For this review, take the finished solid that the model builds, in its own axes (mm). Face numbers are marked on the shaded views. Give positions to 0.01 mm unless a question says otherwise; leave off trailing zeros. Loops run counter-clockwise (first coordinate to the right, second up) from the corner with the lowest first, then second, coordinate; pieces in that order, holes last.
```python
from build123d import *
from OCP.BRepFilletAPI import BRepFilletAPI_MakeChamfer

# Parameters (mm, degrees)
SKETCH1_W            = 68.5
SKETCH1_H            = 64.5
BOSS_EXTRUDE3_DEPTH  = 21
SKETCH3_W            = 60.5
SKETCH3_H            = 60.5
CUT_EXTRUDE1_DEPTH   = 15
SKETCH5_W            = 68.5
SKETCH5_H            = 6
BOSS_EXTRUDE4_DEPTH  = 105
SKETCH10_W           = 10
SKETCH10_H           = 29
BOSS_EXTRUDE5_DEPTH  = 5.5
SKETCH9_W            = 4
SKETCH9_H            = 20
CUT_EXTRUDE2_DEPTH   = 20.5
SKETCH11_W           = 6
SKETCH11_H           = 20
CUT_EXTRUDE3_DEPTH   = 5.5
CHAMFER2_SIZE        = 5.5
CHAMFER2_SIZE_2      = 5
CHAMFER3_SIZE        = 2
SKETCH12_W           = 34.25
SKETCH12_H           = 169.5
CUT_EXTRUDE4_DEPTH   = 50
SKETCH15_R           = 1.5
CUT_EXTRUDE5_DEPTH   = 50
SKETCH16_R           = 1.5
CUT_EXTRUDE6_DEPTH   = 50
SKETCH17_R           = 1.5
CUT_EXTRUDE7_DEPTH   = 50
SKETCH19_W           = 34.25
SKETCH19_H           = 6
BOSS_EXTRUDE6_DEPTH  = 7
SKETCH26_W           = 12
SKETCH26_H           = 9
BOSS_EXTRUDE7_DEPTH  = 30
SKETCH20_R           = 3.75
CUT_EXTRUDE9_DEPTH   = 184.263642057
SKETCH21_W           = 3
SKETCH21_H           = 2.563068229
CUT_EXTRUDE10_DEPTH  = 184.263642057
SKETCH18_R           = 1.5
CUT_EXTRUDE8_DEPTH   = 135
SKETCH24_R           = 4
CUT_EXTRUDE13_DEPTH  = 183.278118544
SKETCH25_W           = 3
SKETCH25_H           = 2.291900756
CUT_EXTRUDE14_DEPTH  = 183.278118544
SKETCH27_R           = 1.75
CUT_EXTRUDE15_DEPTH  = 183.278118544
BOSS_EXTRUDE9_START  = 5
SKETCH30_W           = 8
SKETCH30_H           = 8
SKETCH30_R           = 1.75
BOSS_EXTRUDE9_DEPTH  = 5
SKETCH31_W           = 8
SKETCH31_H           = 8
CUT_EXTRUDE16_DEPTH  = 5
SKETCH32_W           = 19.705511252
SKETCH32_H           = 22.257631466
BOSS_EXTRUDE10_DEPTH = 6
SKETCH33_R           = 1.5
CUT_EXTRUDE17_DEPTH  = 9.74
SKETCH34_R           = 3.75
CUT_EXTRUDE18_DEPTH  = 192.688549475
SKETCH36_R           = 2.5
CUT_EXTRUDE20_DEPTH  = 2
SKETCH39_W           = 3
SKETCH39_H           = 4.259893973
CUT_EXTRUDE22_DEPTH  = 192.688549475
SKETCH41_W           = 12
SKETCH41_H           = 9
BOSS_EXTRUDE11_DEPTH = 30
SKETCH42_R           = 3
CUT_EXTRUDE23_DEPTH  = 3
SKETCH44_W           = 10
SKETCH44_H           = 10
BOSS_EXTRUDE12_DEPTH = 5
SKETCH47_R           = 2.5
CUT_EXTRUDE26_DEPTH  = 3
SKETCH46_W           = 4
SKETCH46_H           = 9
CUT_EXTRUDE27_DEPTH  = 9
CUT_EXTRUDE28_START  = -68.5
SKETCH48_R           = 1.5
CUT_EXTRUDE28_DEPTH  = 68.5


with BuildPart() as part:
    # Sketch1 → Boss-Extrude3 (new body)
    with BuildSketch(Plane(origin=(0, 0, 0), x_dir=(1, 0, 0), z_dir=(0, 1, 0))):
        with Locations((-34.25, 32.25)):
            Rectangle(SKETCH1_W, SKETCH1_H)
    extrude(amount=BOSS_EXTRUDE3_DEPTH)

    # Sketch3 → Cut-Extrude1 (cut)
    with BuildSketch(Plane(origin=(0, 21, 0), x_dir=(1, 0, 0), z_dir=(0, 1, 0))):
        with Locations((-34.25, 34.25)):
            Rectangle(SKETCH3_W, SKETCH3_H)
    extrude(amount=-CUT_EXTRUDE1_DEPTH, mode=Mode.SUBTRACT)

    # Sketch5 → Boss-Extrude4 (add)
    with BuildSketch(Plane(origin=(0, 0, -64.5), x_dir=(-1, 0, 0), z_dir=(0, 0, -1))):
        with Locations((34.25, 3)):
            Rectangle(SKETCH5_W, SKETCH5_H)
    extrude(amount=BOSS_EXTRUDE4_DEPTH)

    # Sketch10 → Boss-Extrude5 (add)
    with BuildSketch(Plane.XZ):
        with Locations((-5, -30)):
            Rectangle(SKETCH10_W, SKETCH10_H)
    extrude(amount=BOSS_EXTRUDE5_DEPTH)

    # Sketch9 → Cut-Extrude2 (cut)
    with BuildSketch(Plane(origin=(0, 21, 0), x_dir=(1, 0, 0), z_dir=(0, 1, 0))):
        with Locations((-2, 28)):
            Rectangle(SKETCH9_W, SKETCH9_H)
    extrude(amount=-CUT_EXTRUDE2_DEPTH, mode=Mode.SUBTRACT)

    # Sketch11 → Cut-Extrude3 (cut)
    with BuildSketch(Plane(origin=(0, 6, 0), x_dir=(1, 0, 0), z_dir=(0, 1, 0))):
        with Locations((-7, 28)):
            Rectangle(SKETCH11_W, SKETCH11_H)
    extrude(amount=-CUT_EXTRUDE3_DEPTH, mode=Mode.SUBTRACT)

    # Chamfer2
    chamfer2_edges_1 = [part.edges().sort_by_distance(p)[0] for p in [
        (-5, -5.5, -44.5),
    ]]
    chamfer2_side_1 = [part.faces().sort_by_distance(p)[0] for p in [
        (-5, -5.4, -44.5),
    ]]
    chamfer2_edges_2 = [part.edges().sort_by_distance(p)[0] for p in [
        (-5, -5.5, -15.5),
    ]]
    chamfer2_side_2 = [part.faces().sort_by_distance(p)[0] for p in [
        (-5, -5.5, -15.6),
    ]]
    chamfer2 = BRepFilletAPI_MakeChamfer(part.part.solid().wrapped)
    for e in chamfer2_edges_1:
        chamfer2.Add(CHAMFER2_SIZE - 0.0001, CHAMFER2_SIZE_2 - 0.0001, e.wrapped, chamfer2_side_1[0].wrapped)
    for e in chamfer2_edges_2:
        chamfer2.Add(CHAMFER2_SIZE_2 - 0.0001, CHAMFER2_SIZE - 0.0001, e.wrapped, chamfer2_side_2[0].wrapped)
    add(Compound.cast(chamfer2.Shape()), mode=Mode.REPLACE)  # a hair under: the kernel refuses the full size

    # Chamfer3
    chamfer3_edges = [part.edges().sort_by_distance(p)[0] for p in [
        (-5, 0.5, -38),
        (-5, 0.5, -18),
    ]]
    chamfer(chamfer3_edges, length=CHAMFER3_SIZE)

    # Sketch12 → Cut-Extrude4 (cut)
    with BuildSketch(Plane(origin=(0, 21, 0), x_dir=(1, 0, 0), z_dir=(0, 1, 0))):
        with Locations((-51.375, 84.75)):
            Rectangle(SKETCH12_W, SKETCH12_H)
    extrude(amount=-CUT_EXTRUDE4_DEPTH, mode=Mode.SUBTRACT)

    # Sketch15 → Cut-Extrude5 (cut)
    with BuildSketch(Plane(origin=(0, 0.5, 0), x_dir=(1, 0, 0), z_dir=(0, 1, 0))):
        with Locations(Location((-5, 31.75713966, 0), (0, 0, 270))):
            Circle(SKETCH15_R)
    extrude(amount=-CUT_EXTRUDE5_DEPTH, mode=Mode.SUBTRACT)

    # Sketch16 → Cut-Extrude6 (cut)
    with BuildSketch(Plane(origin=(0, 6, 0), x_dir=(1, 0, 0), z_dir=(0, 1, 0))):
        with Locations(Location((-6, 6, 0), (0, 0, 270))):
            Circle(SKETCH16_R)
    extrude(amount=-CUT_EXTRUDE6_DEPTH, mode=Mode.SUBTRACT)

    # Sketch17 → Cut-Extrude7 (cut)
    with BuildSketch(Plane(origin=(0, 6, 0), x_dir=(1, 0, 0), z_dir=(0, 1, 0))):
        with Locations(Location((-6, 62.5, 0), (0, 0, 270))):
            Circle(SKETCH17_R)
    extrude(amount=-CUT_EXTRUDE7_DEPTH, mode=Mode.SUBTRACT)

    # Sketch19 → Boss-Extrude6 (add)
    with BuildSketch(Plane(origin=(0, 0, -169.5), x_dir=(-1, 0, 0), z_dir=(0, 0, -1))):
        with Locations((17.125, 3)):
            Rectangle(SKETCH19_W, SKETCH19_H)
    extrude(amount=BOSS_EXTRUDE6_DEPTH)

    # Sketch26 → Boss-Extrude7 (add)
    with BuildSketch(Plane(origin=(0, 6, 0), x_dir=(1, 0, 0), z_dir=(0, 1, 0))):
        with Locations((-6, 69)):
            Rectangle(SKETCH26_W, SKETCH26_H)
    extrude(amount=BOSS_EXTRUDE7_DEPTH)

    # Sketch20 → Cut-Extrude9 (cut, through all)
    with BuildSketch(Plane(origin=(0, 0.5, 0), x_dir=(1, 0, 0), z_dir=(0, 1, 0))):
        with Locations(Location((-5, 25.75713966, 0), (0, 0, 270))):
            Circle(SKETCH20_R)
    extrude(amount=-CUT_EXTRUDE9_DEPTH, mode=Mode.SUBTRACT)

    # Sketch21 → Cut-Extrude10 (cut, through all)
    with BuildSketch(Plane(origin=(0, 0.5, 0), x_dir=(1, 0, 0), z_dir=(0, 1, 0))):
        with Locations((-5, 30.475605546)):
            Rectangle(SKETCH21_W, SKETCH21_H)
    extrude(amount=-CUT_EXTRUDE10_DEPTH, mode=Mode.SUBTRACT)

    # Sketch18 → Cut-Extrude8 (cut)
    with BuildSketch(Plane(origin=(0, 6, 0), x_dir=(1, 0, 0), z_dir=(0, 1, 0))):
        with Locations(Location((-13, 166.75713966, 0), (0, 0, 270))):
            Circle(SKETCH18_R)
    extrude(amount=-CUT_EXTRUDE8_DEPTH, mode=Mode.SUBTRACT)

    # Sketch24 → Cut-Extrude13 (cut, through all)
    with BuildSketch(Plane(origin=(0, 6, 0), x_dir=(1, 0, 0), z_dir=(0, 1, 0))):
        with Locations(Location((-13, 160.75713966, 0), (0, 0, 270))):
            Circle(SKETCH24_R)
    extrude(amount=-CUT_EXTRUDE13_DEPTH, mode=Mode.SUBTRACT)

    # Sketch25 → Cut-Extrude14 (cut, through all)
    with BuildSketch(Plane(origin=(0, 6, 0), x_dir=(1, 0, 0), z_dir=(0, 1, 0))):
        with Locations((-13, 165.611189282)):
            Rectangle(SKETCH25_W, SKETCH25_H)
    extrude(amount=-CUT_EXTRUDE14_DEPTH, mode=Mode.SUBTRACT)

    # Sketch27 → Cut-Extrude15 (cut, through all)
    with BuildSketch(Plane(origin=(0, 6, 0), x_dir=(1, 0, 0), z_dir=(0, 1, 0))):
        with Locations(Location((-3, 77.5, 0), (0, 0, 270))):
            Circle(SKETCH27_R)
        with Locations(Location((-3, 163.5, 0), (0, 0, 270))):
            Circle(SKETCH27_R)
    extrude(amount=-CUT_EXTRUDE15_DEPTH, mode=Mode.SUBTRACT)

    # Sketch30 → Boss-Extrude9 (add)
    # profile 1 of 2: a face of its own
    with BuildSketch(Plane(origin=(0, 6, 0), x_dir=(1, 0, 0), z_dir=(0, 1, 0)).offset(BOSS_EXTRUDE9_START)):
        with Locations((-4, 77.5)):
            Rectangle(SKETCH30_W, SKETCH30_H)
        with Locations(Location((-3, 77.5, 0), (0, 0, 270))):
            Circle(SKETCH30_R, mode=Mode.SUBTRACT)
    # profile 2 of 2: a face of its own
    with BuildSketch(Plane(origin=(0, 6, 0), x_dir=(1, 0, 0), z_dir=(0, 1, 0)).offset(BOSS_EXTRUDE9_START)):
        with Locations((-4, 163.5)):
            Rectangle(SKETCH30_W, SKETCH30_H)
        with Locations(Location((-3, 163.5, 0), (0, 0, 270))):
            Circle(SKETCH30_R, mode=Mode.SUBTRACT)
    extrude(amount=-BOSS_EXTRUDE9_DEPTH)

    # Mirror5: part across plane


with BuildPart() as part_1:
    add(part.part)
    add(part.part.mirror(Plane(origin=(-34.25, 0, 0), x_dir=(0, 0, 1), z_dir=(1, 0, 0))))

    # Sketch31 → Cut-Extrude16 (cut)
    with BuildSketch(Plane(origin=(0, 11, 0), x_dir=(1, 0, 0), z_dir=(0, 1, 0))):
        with Locations((-64.5, 163.5)):
            Rectangle(SKETCH31_W, SKETCH31_H)
    extrude(amount=-CUT_EXTRUDE16_DEPTH, mode=Mode.SUBTRACT)

    # Sketch32 → Boss-Extrude10 (add)
    with BuildSketch(Plane(origin=(0, 6, 0), x_dir=(1, 0, 0), z_dir=(0, 1, 0))):
        with Locations((-58.647244374, 165.371184267)):
            Rectangle(SKETCH32_W, SKETCH32_H)
    extrude(amount=-BOSS_EXTRUDE10_DEPTH)

    # Sketch33 → Cut-Extrude17 (cut)
    with BuildSketch(Plane(origin=(0, 6, 0), x_dir=(1, 0, 0), z_dir=(0, 1, 0))):
        with Locations(Location((-62.5, 166.76, 0), (0, 0, 270))):
            Circle(SKETCH33_R)
    extrude(amount=-CUT_EXTRUDE17_DEPTH, mode=Mode.SUBTRACT)

    # Sketch34 → Cut-Extrude18 (cut, through all)
    with BuildSketch(Plane(origin=(0, 6, 0), x_dir=(1, 0, 0), z_dir=(0, 1, 0))):
        with Locations(Location((-62.5, 160.76, 0), (0, 0, 270))):
            Circle(SKETCH34_R)
    extrude(amount=-CUT_EXTRUDE18_DEPTH, mode=Mode.SUBTRACT)

    # Sketch36 → Cut-Extrude20 (cut)
    with BuildSketch(Plane.XZ):
        with Locations(Location((-3, -77.5, 0), (0, 0, 270))):
            Circle(SKETCH36_R)
        with Locations(Location((-3, -163.5, 0), (0, 0, 270))):
            Circle(SKETCH36_R)
        with Locations(Location((-65.5, -77.5, 0), (0, 0, 270))):
            Circle(SKETCH36_R)
    extrude(amount=-CUT_EXTRUDE20_DEPTH, mode=Mode.SUBTRACT)

    # Sketch39 → Cut-Extrude22 (cut, through all)
    with BuildSketch(Plane(origin=(0, 6, 0), x_dir=(1, 0, 0), z_dir=(0, 1, 0))):
        with Locations((-62.5, 164.630053014)):
            Rectangle(SKETCH39_W, SKETCH39_H)
    extrude(amount=-CUT_EXTRUDE22_DEPTH, mode=Mode.SUBTRACT)

    # Sketch41 → Boss-Extrude11 (add)
    with BuildSketch(Plane(origin=(0, 6, 0), x_dir=(1, 0, 0), z_dir=(0, 1, 0))):
        with Locations((-6, 172)):
            Rectangle(SKETCH41_W, SKETCH41_H)
        with Locations((-62.5, 172)):
            Rectangle(SKETCH41_W, SKETCH41_H)
    extrude(amount=BOSS_EXTRUDE11_DEPTH)

    # Sketch42 → Cut-Extrude23 (cut)
    with BuildSketch(Plane(origin=(0, 6, 0), x_dir=(1, 0, 0), z_dir=(0, 1, 0))):
        with Locations((-62.5, 166.76)):
            Circle(SKETCH42_R)
    extrude(amount=CUT_EXTRUDE23_DEPTH, mode=Mode.SUBTRACT)

    # Sketch44 → Boss-Extrude12 (add)
    with BuildSketch(Plane(origin=(0, 6, 0), x_dir=(1, 0, 0), z_dir=(0, 1, 0))):
        with Locations((-53.5, 128.5)):
            Rectangle(SKETCH44_W, SKETCH44_H)
    extrude(amount=BOSS_EXTRUDE12_DEPTH)

    # Sketch47 → Cut-Extrude26 (cut)
    with BuildSketch(Plane(origin=(0, 6, 0), x_dir=(1, 0, 0), z_dir=(0, 1, 0))):
        with Locations((-13, 166.75713966)):
            Circle(SKETCH47_R)
    extrude(amount=CUT_EXTRUDE26_DEPTH, mode=Mode.SUBTRACT)

    # Sketch46 → Cut-Extrude27 (cut)
    with BuildSketch(Plane(origin=(0, 36, 0), x_dir=(1, 0, 0), z_dir=(0, 1, 0))):
        with Locations((-6, 69)):
            Rectangle(SKETCH46_W, SKETCH46_H)
        with Locations((-62.5, 69)):
            Rectangle(SKETCH46_W, SKETCH46_H)
        with Locations((-62.5, 172)):
            Rectangle(SKETCH46_W, SKETCH46_H)
        with Locations((-6, 172)):
            Rectangle(SKETCH46_W, SKETCH46_H)
    extrude(amount=-CUT_EXTRUDE27_DEPTH, mode=Mode.SUBTRACT)

    # Sketch48 → Cut-Extrude28 (cut)
    with BuildSketch(Plane(origin=(0, 0, 0), x_dir=(0, 0, -1), z_dir=(1, 0, 0)).offset(CUT_EXTRUDE28_START)):
        with Locations((69, 31.5)):
            Circle(SKETCH48_R)
        with Locations((172, 31.5)):
            Circle(SKETCH48_R)
    extrude(amount=CUT_EXTRUDE28_DEPTH, mode=Mode.SUBTRACT)


solid = part_1.part
```
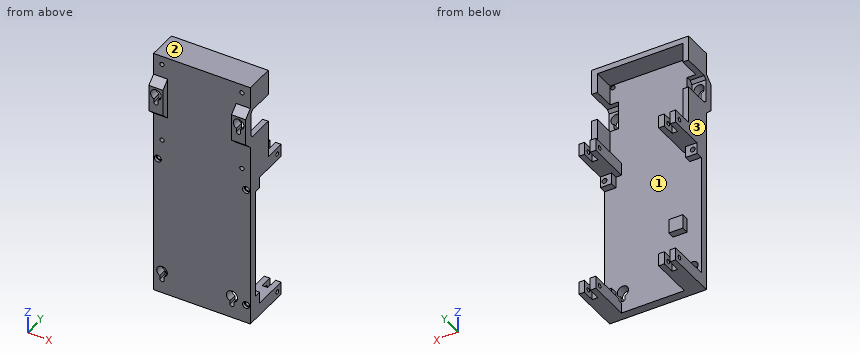
Q1. Consider section A-A on y = -2. Give the boundary of the cut face in (x, z), plus the area to 3 significant figures.
Answers:
outline: (-68.5, -42.68) - (-58.5, -42.68) - (-58.5, -17.32) - (-68.5, -17.32) - close; (-10, -42.68) - (0, -42.68) - (0, -17.32) - (-10, -17.32) - close; hole (-65, -31.76) arc R1.5 ccw to (-62, -31.76) - (-62, -29.19) arc R3.75 ccw (long way) to (-65, -29.19) - close; hole (-6.5, -31.76) arc R1.5 ccw to (-3.5, -31.76) - (-3.5, -29.19) arc R3.75 ccw (long way) to (-6.5, -29.19) - close
area: 398 mm2
Q2. Consider section C-C on z = -88.5. Give the boundary of the cut face in (x, y).
Answers:
outline: (-68.5, 0) - (0, 0) - (0, 6) - (-68.5, 6) - close
Q3. Consider section B-B on x = -50.5. Give the boundary of the cut face in (y, z), plus the area to 3 significant figures.
Answers:
outline: (0, -176.5) - (6, -176.5) - (6, -133.5) - (11, -133.5) - (11, -123.5) - (6, -123.5) - (6, -4) - (21, -4) - (21, 0) - (0, 0) - close
area: 1,170 mm2
Q4. Consider section D-D on x = -21.5. Give the boundary of the cut face in (y, z).
Answers:
outline: (0, -176.5) - (6, -176.5) - (6, -4) - (21, -4) - (21, 0) - (0, 0) - close
Q5. For probe 1 along X at (y, z) = (8, -55); probe 2 along X at (y, z) = (9.5, -79.5); probe 3 along Y at (x, z) = (-66.3, -69), list the stretches that pass through material, from the lowest coordinate up.
Answers:
probe 1: x = -68.5 to -64.5, -4 to 0
probe 2: x = -68.5 to -60.5, -8 to 0
probe 3: y = 0 to 30, 33 to 36
Q6. Mouldability with a two-part tool opening along X and no side actions: class the marked faces 1, 2 and 3 as +X half, -X half, draft (parallel to the pull), parting line (faces both ways), or undercut.
Answers:
face 1: undercut
face 2: draft
face 3: -X half
Q7. For pin 1 Ø4 at (x, z) = (-46.5, -85) entering from -Y; pin 2 Ø6.5 at (x, z) = (-5, -163.5) entering from +Y; pin 3 Ø8 at (x, z) = (-65.5, -28.5) entering from +Y; pin 4 Ø1.5 at (y, z) = (12.5, -159) entering from -X, all flat-tipped, find the tip position at first contact; note any pin that passes through.
Answers:
pin 1: stops at y = 0
pin 2: stops at y = 11
pin 3: stops at y = 0.5
pin 4: passes through
